from build123d import *

# Parameters (mm, degrees)
SKETCH1_R           = 10
BOSS_EXTRUDE1_DEPTH = 7
SKETCH1_3_W         = 7.4
SKETCH1_3_H         = 7.4
BOSS_EXTRUDE2_DEPTH = 7
CHAMFER1_SIZE       = 1
BOSS_EXTRUDE3_START = 1.7
SKETCH1_4_R         = 15
SKETCH1_4_R_2       = 10
BOSS_EXTRUDE3_DEPTH = 1.7


with BuildPart() as part:
    # Sketch1 → Boss-Extrude1 (new body)
    with BuildSketch(Plane.XY):
        Polygon((-30, 0), (-15, -48.118283633), (15, -48.118283633), (30, 0), (13.753072731, 52.118283633), (-13.753072731, 52.118283633), align=None)
        Circle(SKETCH1_R, mode=Mode.SUBTRACT)
    extrude(amount=-BOSS_EXTRUDE1_DEPTH)

    # Sketch1<3> → Boss-Extrude2 (add)
    with BuildSketch(Plane.XY):
        with Locations((-11.25, -29.468283633)):
            Rectangle(SKETCH1_3_W, SKETCH1_3_H)
        with Locations((10.003072731, 33.468283633)):
            Rectangle(SKETCH1_3_W, SKETCH1_3_H)
    extrude(amount=BOSS_EXTRUDE2_DEPTH)

    # Chamfer1
    chamfer1_edges = [part.edges().sort_by_distance(p)[0] for p in [
        (-11.25, -25.768283633, 7),
        (-14.95, -29.468283633, 7),
        (-11.25, -33.168283633, 7),
        (-7.55, -29.468283633, 7),
        (10.003072731, 29.768283633, 7),
        (13.703072731, 33.468283633, 7),
        (10.003072731, 37.168283633, 7),
        (6.303072731, 33.468283633, 7),
    ]]
    chamfer(chamfer1_edges, length=CHAMFER1_SIZE)

    # Sketch1<4> → Boss-Extrude3 (add)
    with BuildSketch(Plane.XY.offset(BOSS_EXTRUDE3_START)):
        Circle(SKETCH1_4_R)
        Circle(SKETCH1_4_R_2, mode=Mode.SUBTRACT)
    extrude(amount=-BOSS_EXTRUDE3_DEPTH)


solid = part.part
Geometry check sheet. Reference: the model listing, model coordinates, mm. A direction names the side the tool comes from. Give positions to 0.01 mm unless a question says otherwise; leave off trailing zeros. Order: outer loops, then holes, each group sorted by start corner. A loop starts at its lowest first (then second) coordinate and runs counter-clockwise, first axis right, second up. Notation, with made-up numbers: (-15.5, 80) - (-11.5, 80) arc R16 cw to (-11.5, 89) - close; hole circle Ø8 at (52, 27.25). An arc over 180 degrees is marked (long way). Answer as a JSON object with one key per item and string values.
(1) Cross-section at C-C (y = 6). Record the cut outline in (x, z), then the cut area to 3 significant figures.
Report:
{"outline": "(-28.13, -7) - (-8, -7) - (-8, 1.7) - (-13.75, 1.7) - (-13.75, 0) - (-28.13, 0) - close; (8, -7) - (28.13, -7) - (28.13, 0) - (13.75, 0) - (13.75, 1.7) - (8, 1.7) - close", "area": "301 mm^2"}
(2) Tool access check on faces 1 (the flat face through (3, -10, 1.7)), 2 (the flat face through (10, 37.168, 3)), 3 (the cylindrical face through (-14.985, 0.66, 0.862)). Record the directions out of +Z, -Z, +X, -X, +Y, -Y that give a thin tool (end or side, any length) a straight path to the whole face; none if there is none.
Report:
{"face 1": "+Z, +X, -X", "face 2": "+Z, +X, -X, +Y", "face 3": "+Z"}
(3) Cross-section at D-D (z = -4). Record the cut outline in (x, y).
Report:
{"outline": "(-30, 0) - (-15, -48.12) - (15, -48.12) - (30, 0) - (13.75, 52.12) - (-13.75, 52.12) - close; hole circle Ø20 at (0, 0)"}
(4) Cross-section at B-B (x = 0). Record the cut outline in (y, z).
Report:
{"outline": "(-48.12, -7) - (-10, -7) - (-10, 1.7) - (-15, 1.7) - (-15, 0) - (-48.12, 0) - close; (10, -7) - (52.12, -7) - (52.12, 0) - (15, 0) - (15, 1.7) - (10, 1.7) - close"}
(5) Depth check by flat-ended pin: pin 1 Ø1.8 at (y, z) = (-30, 3.5) entering from -X; pin 2 Ø4 at (y, z) = (38, 3.5) entering from -X; pin 3 Ø12 at (x, y) = (13.5, 3.5) entering from +Z; pin 4 Ø16 at (x, y) = (0, 0) entering from -Z. Enter the tip coordinate at first touch or a pass-through.
Report:
{"pin 1": "x = -14.95", "pin 2": "x = 6.3", "pin 3": "z = 1.7", "pin 4": "through"}
(6) Cross-section at A-A (z = 3.5). Record the cut outline in (x, y).
Report:
{"outline": "(-14.95, -33.17) - (-7.55, -33.17) - (-7.55, -25.77) - (-14.95, -25.77) - close; (6.3, 29.77) - (13.7, 29.77) - (13.7, 37.17) - (6.3, 37.17) - close"}
(7) Material ranges on line 1 (Y direction, x = 0, z = -4.5); line 2 (Y direction, x = -1.5, z = -5.5); line 3 (Z direction, x = 12, y = -23), recorded low to high.
Report:
{"line 1": "-48.12 to -10, 10 to 52.12", "line 2": "-48.12 to -9.89, 9.89 to 52.12", "line 3": "-7 to 0"}
(8) Draft check along X on faces 4 (the flat face through (13.703, 33, 3)), 5 (the flat face through (6.303, 33, 3)), 6 (the flat face through (0, 52.118, -3)), 7 (the cylindrical face through (-2.17, -9.76, -2.59)). Enter one of: released by +X, released by -X, zero draft, split by the parting line, or undercut.
Report:
{"face 4": "released by +X", "face 5": "released by -X", "face 6": "zero draft", "face 7": "undercut"}
